```python
from build123d import *

# Parameters (mm, degrees)
PLACA_START                        = -10.35
PLACA_DEPTH                        = 6.35
PLACA_R1_START                     = -10.35
CROQUIS2_R                         = 35
PLACA_R1_DEPTH                     = 6.35
PLACA_R2_START                     = -10.35
CROQUIS3_R                         = 30
PLACA_R2_DEPTH                     = 6.35
ALIGERADO_START                    = -10.35
ALIGERADO_DEPTH                    = 6.35
BARRENOS_SEPARADORES_M4_START      = -10.35
CROQUIS5_R                         = 2.25
BARRENOS_SEPARADORES_M4_DEPTH      = 6.35
PASO_PIN_Y_ROSCA_M4_EJEFALSO_START = -10.35
CROQUIS6_R                         = 5.25
CROQUIS6_R_2                       = 3.5
CROQUIS6_R_3                       = 1.65
PASO_PIN_Y_ROSCA_M4_EJEFALSO_DEPTH = 6.35
ROSCA_M3_BASES_CINCHO_START        = -10.35
CROQUIS7_R                         = 1.25
ROSCA_M3_BASES_CINCHO_DEPTH        = 6.35
PASO_M3_BASES_CINCHO_START         = -10.35
CROQUIS8_R                         = 1.7
PASO_M3_BASES_CINCHO_DEPTH         = 6.35
CROQUIS9_R                         = 10
SALIENTE_EXTRUIR1_DEPTH            = 4.5
CROQUIS10_R                        = 7.475
CORTAR_EXTRUIR1_DEPTH              = 10


with BuildPart() as part:
    # Croquis1 → Placa (new body)
    with BuildSketch(Plane(origin=(0, 0, 0), x_dir=(1, 0, 0), z_dir=(0, 1, 0)).offset(PLACA_START)):
        Polygon((1.148293963, -206.431158085), (153.384251969, -201.433849787), (153.384251969, -141.466150213), (1.148293963, -136.468841915), align=None)
    extrude(amount=PLACA_DEPTH)

    # Croquis2 → Placa_r1 (add)
    with BuildSketch(Plane(origin=(0, 0, 0), x_dir=(1, 0, 0), z_dir=(0, 1, 0)).offset(PLACA_R1_START)):
        with Locations((0, -171.45)):
            Circle(CROQUIS2_R)
    extrude(amount=PLACA_R1_DEPTH)

    # Croquis3 → Placa_r2 (add)
    with BuildSketch(Plane(origin=(0, 0, 0), x_dir=(1, 0, 0), z_dir=(0, 1, 0)).offset(PLACA_R2_START)):
        with Locations((152.4, -171.45)):
            Circle(CROQUIS3_R)
    extrude(amount=PLACA_R2_DEPTH)

    # Croquis4 → Aligerado (cut)
    with BuildSketch(Plane(origin=(0, 0, 0), x_dir=(1, 0, 0), z_dir=(0, 1, 0)).offset(ALIGERADO_START)):
        with BuildLine():
            Line((55, -162.45), (75, -162.45))
            ThreePointArc((75, -162.45), (84, -171.45), (75, -180.45))
            Line((75, -180.45), (55, -180.45))
            ThreePointArc((55, -180.45), (46, -171.45), (55, -162.45))
        make_face()
    extrude(amount=ALIGERADO_DEPTH, mode=Mode.SUBTRACT)

    # Croquis5 → Barrenos_separadores_M4 (cut)
    with BuildSketch(Plane(origin=(0, 0, 0), x_dir=(1, 0, 0), z_dir=(0, 1, 0)).offset(BARRENOS_SEPARADORES_M4_START)):
        with Locations(Location((40, -195.45, 0), (0, 0, 270))):
            Circle(CROQUIS5_R)
        with Locations(Location((40, -147.45, 0), (0, 0, 270))):
            Circle(CROQUIS5_R)
        with Locations(Location((90, -191.45, 0), (0, 0, 270))):
            Circle(CROQUIS5_R)
        with Locations(Location((90, -151.45, 0), (0, 0, 270))):
            Circle(CROQUIS5_R)
    extrude(amount=BARRENOS_SEPARADORES_M4_DEPTH, mode=Mode.SUBTRACT)

    # Croquis6 → Paso_pin_y_rosca_M4_ejefalso (cut)
    with BuildSketch(Plane(origin=(0, 0, 0), x_dir=(1, 0, 0), z_dir=(0, 1, 0)).offset(PASO_PIN_Y_ROSCA_M4_EJEFALSO_START)):
        with Locations(Location((0, -171.45, 0), (0, 0, 270))):
            Circle(CROQUIS6_R)
        with Locations(Location((152.4, -171.45, 0), (0, 0, 270))):
            Circle(CROQUIS6_R_2)
        with Locations(Location((152.4, -190.95, 0), (0, 0, 270))):
            Circle(CROQUIS6_R_3)
        with Locations(Location((152.4, -151.95, 0), (0, 0, 270))):
            Circle(CROQUIS6_R_3)
    extrude(amount=PASO_PIN_Y_ROSCA_M4_EJEFALSO_DEPTH, mode=Mode.SUBTRACT)

    # Croquis7 → Rosca_M3_bases_cincho (cut)
    with BuildSketch(Plane(origin=(0, 0, 0), x_dir=(1, 0, 0), z_dir=(0, 1, 0)).offset(ROSCA_M3_BASES_CINCHO_START)):
        with Locations(Location((112, -171.45, 0), (0, 0, 270))):
            Circle(CROQUIS7_R)
    extrude(amount=ROSCA_M3_BASES_CINCHO_DEPTH, mode=Mode.SUBTRACT)

    # Croquis8 → Paso_M3_bases_cincho (cut)
    with BuildSketch(Plane(origin=(0, 0, 0), x_dir=(1, 0, 0), z_dir=(0, 1, 0)).offset(PASO_M3_BASES_CINCHO_START)):
        with Locations(Location((112, -171.45, 0), (0, 0, 270))):
            Circle(CROQUIS8_R)
    extrude(amount=PASO_M3_BASES_CINCHO_DEPTH, mode=Mode.SUBTRACT)

    # Croquis9 → Saliente-Extruir1 (add)
    with BuildSketch(Plane.XZ.offset(10.35)):
        with Locations(Location((0, 171.45, 0), (0, 0, 270))):
            Circle(CROQUIS9_R)
    extrude(amount=SALIENTE_EXTRUIR1_DEPTH)

    # Croquis10 → Cortar-Extruir1 (cut)
    with BuildSketch(Plane.XZ.offset(14.85)):
        with Locations(Location((0, 171.45, 0), (0, 0, 270))):
            Circle(CROQUIS10_R)
    extrude(amount=-CORTAR_EXTRUIR1_DEPTH, mode=Mode.SUBTRACT)


solid = part.part
```
The model under review builds one solid part; all positions refer to its coordinate system, in mm. A direction names the side the tool comes from. Round coordinates to 2 decimals unless told otherwise and drop trailing zeros. Loops run counter-clockwise (first coordinate to the right, second up) from the corner with the lowest first, then second, coordinate; pieces in that order, holes last. Notation, with made-up numbers: M -33.75,66.5 L -18.75,66.5 A20 ccw -18.75,81.5 Z; hole C 41,20 d3. An arc over 180 degrees is marked long. Put each result on its own line as item: value.
Q1. Consider section D-D, the plane z = 156. Give the boundary of the cut face in (x, y).
Result set:
outline: M -31.41,-10.35 L 178.12,-10.35 L 178.12,-4 L -31.41,-4 Z
Q2. Consider section C-C, the plane x = 63. Give the boundary of the cut face in (y, z).
Result set:
outline: M -10.35,138.5 L -4,138.5 L -4,162.45 L -10.35,162.45 Z; M -10.35,180.45 L -4,180.45 L -4,204.4 L -10.35,204.4 Z
Q3. To check wall thickness, follow L1, parallel to X at y = -5.5, z = 171.45 (3 decimals); L2, parallel to X at y = -7.75, z = 151.95; L3, parallel to X at y = -6, z = 151.45. State the ranges of each line that lie inside material, in increasing order.
Result set:
L1: x = -35 to -7.475, 7.475 to 46, 84 to 110.3, 113.7 to 148.9, 155.9 to 182.4
L2: x = -29.06 to 87.81, 92.19 to 150.75, 154.05 to 175.2
L3: x = -28.72 to 87.75, 92.25 to 150.83, 153.97 to 174.76
Q4. Machinability: for faces 1 (the flat face through (-7, -14.85, 168)), 2 (the flat face through (65, -7, 162.45)), 3 (the cylindrical face through (-2.863, -9.92, 164.545)), which of the approach directions +Z, -Z, +X, -X, +Y, -Y give a long, thin tool a straight path to every point of the face, cutting with its end or side? Answer none if there is none.
Result set:
face 1: +Z, -Z, +X, -X, -Y
face 2: +Y, -Y
face 3: -Y
Q5. Consider section B-B, the plane y = -8. Count the separate pieces of the cut face and the enclosed holes in it, then the cut area to 3 significant figures.
Result set:
separate pieces: 1
enclosed holes: 10
area: 12,300 mm²
Q6. Mouldability with a two-part tool opening along Z and no side actions: class faces 4 (the flat face through (65, -7, 180.45)), 5 (the flat face through (72, -10.35, 187)), 6 (the cylindrical face through (-34.99, -7.22, 170.66)) as released by +Z, released by -Z, zero draft, split by the parting line, or undercut.
Result set:
face 4: undercut
face 5: zero draft
face 6: split by the parting line
Q7. For pin 1 (3.5 mm diameter, centred on x = 40, z = 195.45, fed in from +Y); pin 2 (6 mm diameter, centred on x = 129.5, y = -7.5, fed in from +Z); pin 3 (5 mm diameter, centred on x = 63.5, y = -7, fed in from -Z); pin 4 (1 mm diameter, centred on x = 92.5, z = 184, fed in from -Y), all flat-tipped, find the tip position at first contact; note any pin that passes through.
Result set:
pin 1: passes through
pin 2: stops at z = 202.32
pin 3: stops at z = 138.43
pin 4: stops at y = -10.35
Q8. Consider section A-A, the plane x = 40. Give the boundary of the cut face in (y, z).
Result set:
outline: M -10.35,137.74 L -4,137.74 L -4,145.2 L -10.35,145.2 Z; M -10.35,149.7 L -4,149.7 L -4,193.2 L -10.35,193.2 Z; M -10.35,197.7 L -4,197.7 L -4,205.16 L -10.35,205.16 Z
